Input: part model. Units: mm. Frame: model coordinates. A direction names the side the tool comes from. Round coordinates to 2 decimals unless told otherwise and drop trailing zeros. Loops run counter-clockwise (first coordinate to the right, second up) from the corner with the lowest first, then second, coordinate; pieces in that order, holes last. Notation, with made-up numbers: (72.5, -1) -> (84.5, -1) arc R18 cw to (84.5, 8) -> close; hole circle Ø9 at (57, -26). An arc over 180 degrees is marked (long way). Answer as a JSON object with one key per item and string values. Group by question number.
Item 1: Section query A-A on x = -47. Return loops of the section in (y, z), and give its area (3 significant figures).
Item 2: Draft query along X for faces 1 (the flat face through (0, 508, 24)), 2 (the flat face through (-17.96, 507.79, -13.39)), 3 (the flat face through (-28, 0, 0)). Return one class per face: released by +X, released by -X, zero draft, split by the parting line, or undercut.
Item 3: Set-up query: faces 4 (the cylindrical face through (-44.07, 507.79, 13.18)), 5 (the flat face through (-10.14, 507.79, -7.204)), 6 (the flat face through (-17.96, 507.79, 13.39)). Return all of +Z, -Z, +X, -X, +Y, -Y with unobstructed straight access to the full face (end or side cutting, diameter ignored); none if empty.
Item 4: Pin query (flat end, axial travel): pin 1 (6 mm diameter, centred on y = 509, z = -23.5, fed in from -X); pin 2 (8 mm diameter, centred on y = 299.5, z = 6.5, fed in from -X); pin 3 (12 mm diameter, centred on x = -18.5, y = 368, fed in from +Z). Return the tip coordinate at first contact, or that it passes through.
Item 5: Section query B-B on y = 704. Return loops of the section in (x, z).
Item 6: Material intervals for line 1 (X direction, y = 453, z = 0); line 2 (Z direction, x = -47, y = 620.5); line 3 (X direction, y = 961.5, z = -24), sorted ascending. Write a range as [from, to].
Autodesk Inventor part; units mm, degrees
ref_plane "YZ Plane" through (0, 0, 0) normal (1, 0, 0) x (0, 1, 0)
ref_plane "XZ Plane" through (0, 0, 0) normal (0, 1, 0) x (-1, 0, 0)
ref_plane "XY Plane" through (0, 0, 0) normal (0, 0, 1) x (1, 0, 0)
sketch "Sketch1" plane through (0, 0, 0) normal (0, 1, 0) x (-1, 0, 0)
  line L0 (0, 0) -> (0, -37.5)
  line L1 (0, 0) -> (0, 37.5)
  line L2 (0, 37.5) -> (7, 37.5)
  line L3 (7, 37.5) -> (7, 17.5)
  line L4 (0, -37.5) -> (7, -37.5)
  line L5 (7, -37.5) -> (7, -17.5)
  line L6 (7, 0) -> (27, 0) construction
  line L7 (27, -10) -> (7, -17.5)
  line L8 (7, 17.5) -> (27, 10)
  line L9 (27, 0) -> (47, 0)
  circle A0 centre (47, 0) radius 20
  circle A1 centre (47, 0) radius 13.5
  line L10 (27, 10) -> (29.224, 9.166)
  line L11 (27, -10) -> (29.224, -9.166)
  line L12 (0, 17.5) -> (0, 10.5)
  line L13 (20, 0) -> (20, 4)
  line L14 (0, 10.5) -> (20, 4)
  line L15 (0, -17.5) -> (0, -10.5)
  line L16 (20, 0) -> (20, -4)
  line L17 (20, -4) -> (0, -10.5)
  dimension "d0" = 37.5
  dimension "d1" = 37.5
  dimension "d2" = 7
  dimension "d3" = 20
  dimension "d4" = 20
  dimension "d11" = 27
  dimension "d12" = 7
  dimension "d14" = 4
  dimension "d16" = 7
  dimension "d18" = 4
extrude "Extrusion1" add sketch "Sketch1" along normal blind 1030 contours L17 L16 L13 L14 L1 L2 L3 L8 L10 A0 L11 L7 L5 L4 L0 | A0
sketch "Sketch2" plane through (0, 1030, 0) normal (0, 1, 0) x (1, 0, 0)
  point P0 (0, 0)
properties part number "linear_drive_new"
Solved:
{
 "1": {"outline": "(0, -20) -> (1030, -20) -> (1030, -13.5) -> (0, -13.5) -> close; (0, 13.5) -> (1030, 13.5) -> (1030, 20) -> (0, 20) -> close", "area": "13,400 mm²"},
 "2": {"face 1": "released by +X", "face 2": "undercut", "face 3": "zero draft"},
 "3": {"face 4": "+Y, -Y", "face 5": "+X, +Y, -Y", "face 6": "+Z, +Y, -Y"},
 "4": {"pin 1": "x = -7", "pin 2": "x = -66.84", "pin 3": "z = 15.44"},
 "5": {"outline": "(-29.22, -9.17) -> (-7, -17.5) -> (-7, -37.5) -> (0, -37.5) -> (0, -10.5) -> (-20, -4) -> (-20, 4) -> (0, 10.5) -> (0, 37.5) -> (-7, 37.5) -> (-7, 17.5) -> (-29.22, 9.17) arc R20 ccw (long way) to start; hole circle Ø27 at (-47, 0)"},
 "6": {"line 1": "[-67, -60.5], [-33.5, -20]", "line 2": "[-20, -13.5], [13.5, 20]", "line 3": "[-7, 0]"}
}
